Geometry check sheet. Reference: the model listing, model coordinates, mm. A direction names the side the tool comes from. Round coordinates to 2 decimals unless told otherwise and drop trailing zeros. Loops run counter-clockwise (first coordinate to the right, second up) from the corner with the lowest first, then second, coordinate; pieces in that order, holes last. Notation, with made-up numbers: (35, 54.25) -> (91, 54.25) arc R23 cw to (91, 66.25) -> close; hole circle Ø9 at (22, 57). An arc over 180 degrees is marked (long way). Use one line per item in the form item = value.
from build123d import *

# Parameters (mm, degrees)
BOSS_EXTRUDE1_DEPTH = 10
SKETCH2_R           = 1.775
CUT_EXTRUDE1_DEPTH  = 68.967856728
SKETCH3_R           = 1.775
CUT_EXTRUDE2_DEPTH  = 68.967856728
SKETCH4_W           = 1.25
SKETCH4_H           = 14
SKETCH4_W_2         = 2.106329952
CUT_EXTRUDE3_DEPTH  = 68.967856728


with BuildPart() as part:
    # Sketch1 → Boss-Extrude1 (new body)
    with BuildSketch(Plane(origin=(0, 0, 0), x_dir=(1, 0, 0), z_dir=(0, 1, 0))):
        Polygon((-4, 64.77367944), (4, 64.77367944), (4, 22.77367944), (18, 22.77367944), (18, -9.22632056), (12, -9.22632056), (12, 14.77367944), (-12, 14.77367944), (-12, -9.22632056), (-18, -9.22632056), (-18, 22.77367944), (-4, 22.77367944), align=None)
    extrude(amount=BOSS_EXTRUDE1_DEPTH)

    # Sketch2 → Cut-Extrude1 (cut, through all)
    with BuildSketch(Plane(origin=(0, 10, 0), x_dir=(1, 0, 0), z_dir=(0, 1, 0))):
        with Locations(Location((0, 44.77367944, 0), (0, 0, 270))):
            Circle(SKETCH2_R)
        with Locations(Location((0, 59.77367944, 0), (0, 0, 270))):
            Circle(SKETCH2_R)
    extrude(amount=-CUT_EXTRUDE1_DEPTH, mode=Mode.SUBTRACT)

    # Sketch3 → Cut-Extrude2 (cut, through all)
    with BuildSketch(Plane(origin=(0, 10, 0), x_dir=(1, 0, 0), z_dir=(0, 1, 0))):
        with Locations(Location((-15.2, -4.855416268, 0), (0, 0, 270))):
            Circle(SKETCH3_R)
        with Locations(Location((15.2, -4.855416268, 0), (0, 0, 270))):
            Circle(SKETCH3_R)
        with Locations(Location((-15.2, 19.144583732, 0), (0, 0, 270))):
            Circle(SKETCH3_R)
        with Locations(Location((15.2, 19.144583732, 0), (0, 0, 270))):
            Circle(SKETCH3_R)
    extrude(amount=-CUT_EXTRUDE2_DEPTH, mode=Mode.SUBTRACT)

    # Sketch4 → Cut-Extrude3 (cut, through all)
    with BuildSketch(Plane(origin=(0, 10, 0), x_dir=(1, 0, 0), z_dir=(0, 1, 0))):
        with Locations((-12.625, 5.77367944)):
            Rectangle(SKETCH4_W, SKETCH4_H)
        with Locations((13.053164976, 5.77367944)):
            Rectangle(SKETCH4_W_2, SKETCH4_H)
    extrude(amount=-CUT_EXTRUDE3_DEPTH, mode=Mode.SUBTRACT)


solid = part.part
1. Material ranges on line 1 along X through (y, z) = (8.25, -4); line 2 along Z through (x, y) = (-15.5, 0.75); line 3 along X through (y, z) = (2, -52), recorded low to high.
Return value:
line_1 = -18 to -13.25, 14.11 to 18
line_2 = -22.77 to -20.89, -17.4 to 3.11, 6.6 to 9.23
line_3 = -4 to 4
2. Section check C-C (y = 5.25). Record the boundary of the cut face in (x, z) (3 decimals), then the cut area to 3 significant figures.
Return value:
outline = (-18, -22.774) -> (-4, -22.774) -> (-4, -64.774) -> (4, -64.774) -> (4, -22.774) -> (18, -22.774) -> (18, 9.226) -> (12, 9.226) -> (12, 1.226) -> (14.106, 1.226) -> (14.106, -12.774) -> (12, -12.774) -> (12, -14.774) -> (-12, -14.774) -> (-12, -12.774) -> (-13.25, -12.774) -> (-13.25, 1.226) -> (-12, 1.226) -> (-12, 9.226) -> (-18, 9.226) -> close; hole circle Ø3.55 at (-15.2, -19.145); hole circle Ø3.55 at (-15.2, 4.855); hole circle Ø3.55 at (0, -59.774); hole circle Ø3.55 at (0, -44.774); hole circle Ø3.55 at (15.2, -19.145); hole circle Ø3.55 at (15.2, 4.855)
area = 806 mm2
3. Section check A-A (x = 0). Record the boundary of the cut face in (y, z).
Return value:
outline = (0, -64.77) -> (10, -64.77) -> (10, -61.55) -> (0, -61.55) -> close; (0, -58) -> (10, -58) -> (10, -46.55) -> (0, -46.55) -> close; (0, -43) -> (10, -43) -> (10, -14.77) -> (0, -14.77) -> close
4. Tool access check on faces 5 (the flat face through (0, 5, -14.774)), 6 (the flat face through (11, 5, -22.774)), 7 (the flat face through (0, 5, -64.774)), 8 (the flat face through (-11, 5, -22.774)), 9 (the flat face through (-13.25, 5, -6)). Record the directions out of +Z, -Z, +X, -X, +Y, -Y that give a thin tool (end or side, any length) a straight path to the whole face; none if there is none.
Return value:
face_5 = +Z, +Y, -Y
face_6 = -Z, +X, +Y, -Y
face_7 = -Z, +X, -X, +Y, -Y
face_8 = -Z, -X, +Y, -Y
face_9 = +Y, -Y
5. Mould release check, pull along X, two halves, no side actions. Record for faces 1 (the flat face through (18, 5, -7)), 2 (the cylindrical face through (-15.122, 5.07, -20.918)), 3 (the flat face through (-13, 5, -12.774)), 4 (the flat face through (1, 10, -22)): released by +X, released by -X, zero draft, split by the parting line, or undercut.
Return value:
face_1 = released by +X
face_2 = undercut
face_3 = undercut
face_4 = zero draft
6. Gauge pin test, flat ends, axial feed: pin 1 (0.6 mm diameter, centred on x = 12.5, y = 5.5, fed in from -Z); pin 2 (3 mm diameter, centred on x = -9.5, y = 7, fed in from +Z); pin 3 (1.5 mm diameter, centred on y = 8.5, z = -41, fed in from -X); pin 4 (3 mm diameter, centred on x = -15.2, z = -19.14, fed in from +Y). Record the tip position at first contact, or that the pin passes through.
Return value:
pin_1 = -22.77
pin_2 = -14.77
pin_3 = -4
pin_4 = through
7. Section check D-D (x = -15.2). Record the boundary of the cut face in (y, z), then the cut area to 3 significant figures.
Return value:
outline = (0, -22.77) -> (10, -22.77) -> (10, -20.92) -> (0, -20.92) -> close; (0, -17.37) -> (10, -17.37) -> (10, 3.08) -> (0, 3.08) -> close; (0, 6.63) -> (10, 6.63) -> (10, 9.23) -> (0, 9.23) -> close
area = 249 mm2
8. Section check B-B (z = -0.5). Record the boundary of the cut face in (x, y), then the cut area to 3 significant figures.
Return value:
outline = (-18, 0) -> (-13.25, 0) -> (-13.25, 10) -> (-18, 10) -> close; (14.11, 0) -> (18, 0) -> (18, 10) -> (14.11, 10) -> close
area = 86.4 mm2
